Design review of the part built by this model. Coordinates are the model's own, in mm. Round coordinates to 2 decimals unless told otherwise and drop trailing zeros. Loops run counter-clockwise (first coordinate to the right, second up) from the corner with the lowest first, then second, coordinate; pieces in that order, holes last. Notation, with made-up numbers: M 5,20 L 16,20 A33 cw 16,50 Z; hole C -39,-6 d11. An arc over 180 degrees is marked long. One line per item, written item: value. Start each with the question number.
Item 1: For line 1 along Y through (x, z) = (14.5, 2), list the stretches that pass through material, from the lowest coordinate up.
Item 2: We need section A-A (z = 1.05). Write out the cut boundary in (x, y), then the cut area to 3 significant figures.
Item 3: We need section B-B (x = 13.5). Write out the cut boundary in (y, z).
Item 4: Clearance check with flat-ended pins moving along their axes: pin 1 (0.8 mm diameter, centred on y = -1.5, z = 1.5, fed in from +X); pin 2 (2 mm diameter, centred on x = 3, y = 52, fed in from -Z); pin 3 (1.5 mm diameter, centred on x = 14, z = 1, fed in from +Y); pin 4 (0.9 mm diameter, centred on x = 13.5, z = 1.5, fed in from -Y). State where each tip first meets the part, or that it passes through.
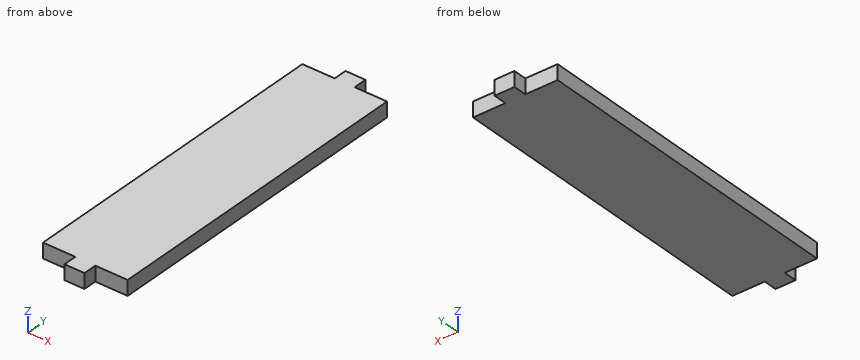
Autodesk Inventor part; units mm, degrees
ref_plane "YZ Plane" through (0, 0, 0) normal (1, 0, 0) x (0, 1, 0)
ref_plane "XZ Plane" through (0, 0, 0) normal (0, 1, 0) x (-1, 0, 0)
ref_plane "XY Plane" through (0, 0, 0) normal (0, 0, 1) x (1, 0, 0)
sketch "Sketch3" plane through (0, 0, 0) normal (0, 0, 1) x (1, 0, 0)
  line L0 (0, 0) -> (17, 0)
  line L1 (17, 0) -> (17, 65)
  line L2 (17, 65) -> (0, 65)
  line L3 (0, 65) -> (0, 0)
  dimension "d0" = 17
  dimension "d1" = 65
  dimension "d2" = 17
extrude "Extrusion1" add sketch "Sketch3" along normal blind 3
sketch "Sketch4" plane through (0, 0, 0) normal (0, -1, 0) x (1, 0, 0)
  line L0 (0, 0) -> (0, 3)
  line L1 (0, 1.5) -> (17, 1.5)
  line L2 (17, 0) -> (17, 3)
  line L3 (17, 3) -> (0, 3)
  line L4 (8.5, 3) -> (8.5, 0)
  line L5 (17, 0) -> (0, 0)
  line L6 (8.5, 1.5) -> (6.5, 1.5)
  line L7 (6.5, 1.5) -> (6.5, 3)
  line L8 (8.5, 1.5) -> (10.5, 1.5)
  line L9 (10.5, 1.5) -> (10.5, 0)
  line L10 (6.5, 3) -> (10.5, 3)
  line L11 (10.5, 3) -> (10.5, 0)
  line L12 (10.5, 0) -> (6.5, 0)
  line L13 (6.5, 0) -> (6.5, 3)
  dimension "d5" = 2
  dimension "d6" = 1.5
  dimension "d7" = 2
  dimension "d8" = 1.5
extrude "Extrusion2" add sketch "Sketch4" along normal blind 2.7 contours L13 L1 L4 L5 | L7 L3 L4 L1 | L4 L1 L9 L5 | L4 L3 L11 L1
extrude "Extrusion3" add sketch "Sketch4" against normal blind 2.7 from surface at -65 contours L13 L1 L4 L5 | L7 L3 L4 L1 | L4 L1 L9 L5 | L4 L3 L11 L1
properties part number "carcasa_piezasRadio_3.0"
A:
1. line 1: 0 to 65
2. outline: M 0,0 L 6.5,0 L 6.5,-2.7 L 10.5,-2.7 L 10.5,0 L 17,0 L 17,65 L 10.5,65 L 10.5,67.7 L 6.5,67.7 L 6.5,65 L 0,65 Z
2. area: 1,130 mm2
3. outline: M 0,0 L 65,0 L 65,3 L 0,3 Z
4. pin 1: x = 10.5
4. pin 2: z = 0
4. pin 3: y = 65
4. pin 4: y = 0
